```python
from build123d import *

# Parameters (mm, degrees)
SKETCH1_R                       = 80.518
SKETCH1_R_2                     = 79.375
BOSS_EXTRUDE1_DEPTH             = 817.5625
TAP_DRILL_FOR_10_32_TAP1_REACH  = 839.152
TAP_DRILL_FOR_10_32_TAP1_BORE_R = 2.0193
TAP_DRILL_FOR_4_40_TAP1_REACH   = 839.152
TAP_DRILL_FOR_4_40_TAP1_BORE_R  = 1.1303
CIRPATTERN1_COUNT               = 6


with BuildPart() as part:
    # Sketch1 → Boss-Extrude1 (new body)
    with BuildSketch(Plane.XY):
        Circle(SKETCH1_R)
        Circle(SKETCH1_R_2, mode=Mode.SUBTRACT)
    extrude(amount=BOSS_EXTRUDE1_DEPTH)

    # Tap Drill for #10-32 Tap1 bore → Tap Drill for #10-32 Tap1 (cut, up to next)
    with BuildSketch(Plane(origin=(0, 80.518, 0), x_dir=(1, 0, 0), z_dir=(0, 1, 0)), mode=Mode.PRIVATE) as tap_drill_for_10_32_tap1_sk1:
        with Locations((0, -76.2)):
            Circle(TAP_DRILL_FOR_10_32_TAP1_BORE_R)
    tap_drill_for_10_32_tap1_tool1 = extrude(tap_drill_for_10_32_tap1_sk1.sketch, amount=-TAP_DRILL_FOR_10_32_TAP1_REACH, mode=Mode.PRIVATE) & part.part
    tap_drill_for_10_32_tap1 = tap_drill_for_10_32_tap1_tool1.solids().sort_by_distance((0, 80.518, 76.2))[0]
    add(tap_drill_for_10_32_tap1, mode=Mode.SUBTRACT)

    # Tap Drill for #4-40 Tap1 bore → Tap Drill for #4-40 Tap1 (cut, up to next)
    with BuildSketch(Plane(origin=(0, 80.518, 0), x_dir=(1, 0, 0), z_dir=(0, 1, 0)), mode=Mode.PRIVATE) as tap_drill_for_4_40_tap1_sk1:
        with Locations((0, -738.1875)):
            Circle(TAP_DRILL_FOR_4_40_TAP1_BORE_R)
    tap_drill_for_4_40_tap1_tool1 = extrude(tap_drill_for_4_40_tap1_sk1.sketch, amount=-TAP_DRILL_FOR_4_40_TAP1_REACH, mode=Mode.PRIVATE) & part.part
    tap_drill_for_4_40_tap1 = tap_drill_for_4_40_tap1_tool1.solids().sort_by_distance((0, 80.518, 738.1875))[0]
    add(tap_drill_for_4_40_tap1, mode=Mode.SUBTRACT)

    # CirPattern1: Tap Drill for #10-32 Tap1, Tap Drill for #4-40 Tap1 ×6 about axis
    cirpattern1_axis = Axis((0, 0, 817.5625), (0, 0, 1))
    add([tap_drill_for_10_32_tap1.rotate(cirpattern1_axis, i * 360 / CIRPATTERN1_COUNT) for i in range(1, CIRPATTERN1_COUNT)], mode=Mode.SUBTRACT)
    add([tap_drill_for_4_40_tap1.rotate(cirpattern1_axis, i * 360 / CIRPATTERN1_COUNT) for i in range(1, CIRPATTERN1_COUNT)], mode=Mode.SUBTRACT)


solid = part.part
```
Geometry: final body of the model. Coordinates: model frame, mm. Round coordinates to 2 decimals unless told otherwise and drop trailing zeros. Order: outer loops, then holes, each group sorted by start corner. A loop starts at its lowest first (then second) coordinate and runs counter-clockwise, first axis right, second up. Notation, with made-up numbers: M -5.75,-12 L 5.25,-12 A22 ccw 5.25,18 Z; hole C -3,8 d9. An arc over 180 degrees is marked long. Use one line per item in the form item = value. Start each with the question number.
Q1. Pin query (flat end, axial travel): pin 1 Ø10 at (y, z) = (-55.5, 257) entering from +X; pin 2 Ø3 at (y, z) = (17.5, 333) entering from -X; pin 3 Ø1.5 at (x, z) = (-58, 240.5) entering from -Y. Return the tip coordinate at first contact, or that it passes through.
Q2. Cut plane C-C (z = 334). Return loops of the section in (x, y) (3 decimals).
Q3. Mould query, pull axis Y, two halves, no side actions, for faces 1 (the face through (59.3, -53.3, 817.562)), 2 (the face through (-59.345, 54.418, 403.058)), 3 (the face through (75.71, 23.84, 403.06)). Classes: +Y half, -Y half, draft (parallel to the pull), parting line (faces both ways), or undercut.
Q4. Cut plane B-B (x = -53.5). Return loops of the section in (y, z).
Q5. Material intervals for line 1 (Z direction, x = 0, y = 79.7); line 2 (X direction, y = 3, z = 159.5); line 3 (Y direction, x = 0, z = 574) (3 decimals), sorted ascending. Write a range as [from, to].
Q6. Cut plane A-A (y = 0). Return loops of the section in (x, z) (1 decimal).
Geometry results:
q1.pin_1 = 62.71
q1.pin_2 = -78.91
q1.pin_3 = -56.62
q2.outline = C 0,0 d161.036; hole C 0,0 d158.75
q3.face_1 = draft
q3.face_2 = parting line
q3.face_3 = undercut
q4.outline = M -60.17,0 L -58.64,0 L -58.64,817.56 L -60.17,817.56 Z; M 58.64,0 L 60.17,0 L 60.17,817.56 L 58.64,817.56 Z
q5.line_1 = [0, 74.18], [78.22, 737.06], [739.32, 817.56]
q5.line_2 = [-80.46, -79.32], [79.32, 80.46]
q5.line_3 = [-80.518, -79.375], [79.375, 80.518]
q6.outline = M -80.5,0 L -79.4,0 L -79.4,817.6 L -80.5,817.6 Z; M 79.4,0 L 80.5,0 L 80.5,817.6 L 79.4,817.6 Z
